```python
from build123d import *

# Parameters (mm, degrees)
SKETCH_2_W                  = 47
SKETCH_2_H                  = 47
EXTRUDE_1_DEPTH             = 4
SKETCH_3_W                  = 47
SKETCH_3_H                  = 2
EXTRUDE_2_DEPTH             = 43
SKETCH_4_W                  = 4
SKETCH_4_H                  = 45
EXTRUDE_3_DEPTH             = 43
SKETCH_5_R                  = 12.5
CUT_EXTRUDE_1_DEPTH         = 81.268300094
M3X0_5_2_D                  = 3
HOLE_WIZARD_M5_1_AT_2_COUNT = 2
HOLE_WIZARD_M5_1_AT_2_PITCH = 14.142135624
HOLE_WIZARD_M5_1_AT_3_COUNT = 2
HOLE_WIZARD_M5_1_AT_3_PITCH = 20
HOLE_WIZARD_M5_1_AT_4_COUNT = 2
HOLE_WIZARD_M5_1_AT_4_PITCH = 14.142135624
EXTRUDE_6_DEPTH             = 45
EXTRUDE_7_DEPTH             = 45
SKETCH_23_W                 = 67
SKETCH_23_H                 = 47
SKETCH_23_R                 = 3.5
SKETCH_23_R_2               = 12.5
EXTRUDE_10_DEPTH            = 3
M2X0_4_1_D                  = 2
SKETCH_27_W                 = 47
SKETCH_27_H                 = 1
CUT_EXTRUDE_2_DEPTH         = 20
FILLET_1_R                  = 2.5
FILLET_2_R                  = 4
SKETCH_29_W                 = 47
SKETCH_29_H                 = 2
EXTRUDE_11_DEPTH            = 20
FILLET_5_R                  = 4
FILLET_6_R                  = 3
M2X0_4_2_D                  = 2
SKETCH_34_W                 = 20
SKETCH_34_H                 = 47
CUT_EXTRUDE_5_DEPTH         = 20
FILLET_7_R                  = 4


with BuildPart() as part:
    # ｽｹｯﾁ2 → ﾎﾞｽ - 押し出し1 (new body)
    with BuildSketch(Plane.XY):
        with Locations((23.5, 23.5)):
            Rectangle(SKETCH_2_W, SKETCH_2_H)
    extrude(amount=EXTRUDE_1_DEPTH)

    # ｽｹｯﾁ3 → ﾎﾞｽ - 押し出し2 (add)
    with BuildSketch(Plane.XY.offset(4)):
        with Locations((23.5, 46)):
            Rectangle(SKETCH_3_W, SKETCH_3_H)
    extrude(amount=EXTRUDE_2_DEPTH)

    # ｽｹｯﾁ4 → ﾎﾞｽ - 押し出し3 (add)
    with BuildSketch(Plane.XY.offset(4)):
        with Locations((45, 22.5)):
            Rectangle(SKETCH_4_W, SKETCH_4_H)
    extrude(amount=EXTRUDE_3_DEPTH)

    # ｽｹｯﾁ5 → ｶｯﾄ - 押し出し1 (cut, through all)
    with BuildSketch(Plane.XZ.offset(-45)):
        with Locations(Location((21.5, 25.5, 0), (0, 0, 270))):
            Circle(SKETCH_5_R)
    extrude(amount=-CUT_EXTRUDE_1_DEPTH, mode=Mode.SUBTRACT)

    # M3x0.5 ねじ穴2 (through all)
    with Locations(Plane(origin=(0, 47, 0), x_dir=(1, 0, 0), z_dir=(0, 1, 0))):
        with Locations((6, -10), (37, -10), (37, -41), (6, -41)):
            Hole(M3X0_5_2_D / 2)

    # ｽｹｯﾁ14 → M5 平皿頭ねじ用皿穴1 (revolve, cut)
    with BuildSketch(Plane(origin=(11.5, 22, 4), x_dir=(0, -1, 0), z_dir=(1, 0, 0))):
        Polygon((0, 0), (0, 4), (2.75, 4), (2.75, 2.45), (5.2, 0), align=None)
    hole_wizard_m5_1 = revolve(axis=Axis((11.5, 22, 10.35), (0, 0, -1)), mode=Mode.SUBTRACT)

    # M5 平皿頭ねじ用皿穴1 at 2: M5 平皿頭ねじ用皿穴1 ×2
    with Locations(*[Vector(0.7071067811865475, 0.7071067811865476, 0) * (i * HOLE_WIZARD_M5_1_AT_2_PITCH) for i in range(1, HOLE_WIZARD_M5_1_AT_2_COUNT)]):
        add(hole_wizard_m5_1, mode=Mode.SUBTRACT)

    # M5 平皿頭ねじ用皿穴1 at 3: M5 平皿頭ねじ用皿穴1 ×2
    with Locations(*[(i * HOLE_WIZARD_M5_1_AT_3_PITCH, 0, 0) for i in range(1, HOLE_WIZARD_M5_1_AT_3_COUNT)]):
        add(hole_wizard_m5_1, mode=Mode.SUBTRACT)

    # M5 平皿頭ねじ用皿穴1 at 4: M5 平皿頭ねじ用皿穴1 ×2
    with Locations(*[Vector(0.7071067811865474, -0.7071067811865478, 0) * (i * HOLE_WIZARD_M5_1_AT_4_PITCH) for i in range(1, HOLE_WIZARD_M5_1_AT_4_COUNT)]):
        add(hole_wizard_m5_1, mode=Mode.SUBTRACT)

    # ｽｹｯﾁ17 → ﾎﾞｽ - 押し出し6 (add)
    with BuildSketch(Plane.XZ.offset(-45)):
        Polygon((43, 4), (39.5, 4), (43, 7.5), align=None)
    extrude(amount=EXTRUDE_6_DEPTH)

    # ｽｹｯﾁ19 → ﾎﾞｽ - 押し出し7 (add)
    with BuildSketch(Plane.XZ.offset(-45)):
        Polygon((0, 4), (3.5, 4), (0, 7.5), align=None)
    extrude(amount=EXTRUDE_7_DEPTH)

    # ｽｹｯﾁ23 → ﾎﾞｽ - 押し出し10 (add)
    with BuildSketch(Plane(origin=(0, 47, 0), x_dir=(1, 0, 0), z_dir=(0, 1, 0))):
        with Locations((13.5, -23.5)):
            Rectangle(SKETCH_23_W, SKETCH_23_H)
        with Locations(Location((6, -10, 0), (0, 0, 270))):
            Circle(SKETCH_23_R, mode=Mode.SUBTRACT)
        with Locations(Location((6, -41, 0), (0, 0, 270))):
            Circle(SKETCH_23_R, mode=Mode.SUBTRACT)
        with Locations(Location((37, -10, 0), (0, 0, 270))):
            Circle(SKETCH_23_R, mode=Mode.SUBTRACT)
        with Locations(Location((37, -41, 0), (0, 0, 270))):
            Circle(SKETCH_23_R, mode=Mode.SUBTRACT)
        with Locations(Location((21.5, -25.5, 0), (0, 0, 90))):
            Circle(SKETCH_23_R_2, mode=Mode.SUBTRACT)
    extrude(amount=EXTRUDE_10_DEPTH)

    # M2x0.4 ねじ穴1 (through all)
    with Locations(Plane(origin=(0, 50, 0), x_dir=(1, 0, 0), z_dir=(0, 1, 0))):
        with Locations((-5, -18), (-14.5, -18)):
            Hole(M2X0_4_1_D / 2)

    # ｽｹｯﾁ27 → ｶｯﾄ - 押し出し2 (cut)
    with BuildSketch(Plane.ZY.offset(20)):
        with Locations((23.5, 47.5)):
            Rectangle(SKETCH_27_W, SKETCH_27_H)
    extrude(amount=-CUT_EXTRUDE_2_DEPTH, mode=Mode.SUBTRACT)

    # ﾌｨﾚｯﾄ1
    fillet_1_edges = [part.edges().sort_by_distance(p)[0] for p in [
        (0, 48, 23.5),
    ]]
    fillet(fillet_1_edges, radius=FILLET_1_R)

    # ﾌｨﾚｯﾄ2
    fillet_2_edges = [part.edges().sort_by_distance(p)[0] for p in [
        (-20, 49, 47),
        (-20, 49, 0),
        (0, 0, 3.75),
        (45, 0, 47),
    ]]
    fillet(fillet_2_edges, radius=FILLET_2_R)

    # ｽｹｯﾁ29 → ﾎﾞｽ - 押し出し11 (add)
    with BuildSketch(Plane(origin=(47, 0, 0), x_dir=(0, 0, -1), z_dir=(1, 0, 0))):
        with Locations((-23.5, 49)):
            Rectangle(SKETCH_29_W, SKETCH_29_H)
    extrude(amount=EXTRUDE_11_DEPTH)

    # ﾌｨﾚｯﾄ5
    fillet_5_edges = [part.edges().sort_by_distance(p)[0] for p in [
        (67, 49, 0),
        (67, 49, 47),
    ]]
    fillet(fillet_5_edges, radius=FILLET_5_R)

    # ﾌｨﾚｯﾄ6
    fillet_6_edges = [part.edges().sort_by_distance(p)[0] for p in [
        (47, 48, 23.5),
    ]]
    fillet(fillet_6_edges, radius=FILLET_6_R)

    # M2x0.4 ねじ穴2 (through all)
    with Locations(Plane(origin=(0, 50, 0), x_dir=(1, 0, 0), z_dir=(0, 1, 0))):
        with Locations((61.5, -18), (52, -18)):
            Hole(M2X0_4_2_D / 2)

    # ｽｹｯﾁ34 → ｶｯﾄ - 押し出し5 (cut)
    with BuildSketch(Plane(origin=(0, 50, 0), x_dir=(1, 0, 0), z_dir=(0, 1, 0))):
        with Locations((-10, -23.5)):
            Rectangle(SKETCH_34_W, SKETCH_34_H)
    extrude(amount=-CUT_EXTRUDE_5_DEPTH, mode=Mode.SUBTRACT)

    # ﾌｨﾚｯﾄ7
    fillet_7_edges = [part.edges().sort_by_distance(p)[0] for p in [
        (0, 47.5, 47),
    ]]
    fillet(fillet_7_edges, radius=FILLET_7_R)


solid = part.part
```
The model under review builds one solid part; all positions refer to its coordinate system, in mm. A direction names the side the tool comes from. Round coordinates to 2 decimals unless told otherwise and drop trailing zeros. Write each loop counter-clockwise with the first axis right and the second up, starting at its lowest first coordinate (ties: lowest second). Pieces come first, ordered by that corner, then holes.
(1) We need section C-C on y = 22. Give the boundary of the cut face in (x, z), and give its area (3 significant figures).
(2) Insertion check: pin 1 (10 mm diameter, centred on x = 32, y = 14.5, fed in from +Z); pin 2 (8 mm diameter, centred on y = 34.5, z = 10.5, fed in from +X); pin 3 (2 mm diameter, centred on x = 6.5, z = 10.5, fed in from +Y); pin 4 (4.5 mm diameter, centred on x = 11.5, y = 22, fed in from +Z). Each pin has a flat end and moves straight along its axis. Give the tip position at first contact, or say it passes through.
(3) We need section B-B on x = 31.5. Give the boundary of the cut face in (y, z).
(4) We need section A-A on z = 25. Give the boundary of the cut face in (x, y), and give its area (3 significant figures).
(5) We need section D-D on z = 10. Give the boundary of the cut face in (x, y), and give its area (3 significant figures).
(6) Mouldability with a two-part tool opening along X and no side actions: class faces 1 (the conical face through (14.33, 22.63, 1.7)), 2 (the flat face through (43, 22, 27)), 3 (the cylindrical face through (65.797, 49.014, 45.859)) as +X half, -X half, draft (parallel to the pull), parting line (faces both ways), or undercut.
(7) Machinability: for faces 4 (the flat face through (21, 23, 4)), 5 (the flat face through (37, 47, 12)), 6 (the conical face through (28.621, 22.378, 1.703)), which of the approach directions +Z, -Z, +X, -X, +Y, -Y give a long, thin tool a straight path to every point of the face, cutting with its end or side? Answer none if there is none.
(8) Wall thickness on L1, parallel to Z at x = 6, y = 45.95; L2, parallel to X at y = 46.5, z = 41; L3, parallel to X at y = 5.5, z = 5: over which ranges is each line inside the solid? List them lowest first.
Findings below:
1. outline: (0, 0) - (8.75, 0) - (8.75, 1.55) - (6.3, 4) - (3.5, 4) - (0, 7.5) - close; (14.25, 0) - (28.75, 0) - (28.75, 1.55) - (26.3, 4) - (16.7, 4) - (14.25, 1.55) - close; (34.25, 0) - (47, 0) - (47, 47) - (43, 47) - (43, 7.5) - (39.5, 4) - (36.7, 4) - (34.25, 1.55) - close
1. area: 316 mm2
2. pin 1: stops at z = 4
2. pin 2: stops at x = 47
2. pin 3: stops at y = 47
2. pin 4: passes through
3. outline: (0, 0) - (19.25, 0) - (19.25, 1.55) - (16.8, 4) - (0, 4) - close; (24.75, 0) - (50, 0) - (50, 18) - (45, 18) - (45, 4) - (27.2, 4) - (24.75, 1.55) - close; (45, 33) - (50, 33) - (50, 47) - (45, 47) - close
4. outline: (0, 45) - (9.01, 45) - (9.01, 50) - (0, 50) - close; (33.99, 45) - (43, 45) - (43, 0) - (47, 0) - (47, 45) arc R3 cw to (50, 48) - (67, 48) - (67, 50) - (33.99, 50) - close
4. area: 332 mm2
5. outline: (0, 45) - (4.5, 45) - (4.5, 47) - (2.5, 47) - (2.5, 50) - (0, 50) - close; (7.5, 45) - (35.5, 45) - (35.5, 47) - (33.5, 47) - (33.5, 50) - (9.5, 50) - (9.5, 47) - (7.5, 47) - close; (38.5, 45) - (43, 45) - (43, 0) - (47, 0) - (47, 45) arc R3 cw to (50, 48) - (67, 48) - (67, 50) - (40.5, 50) - (40.5, 47) - (38.5, 47) - close
5. area: 403 mm2
6. face 1: undercut
6. face 2: -X half
6. face 3: +X half
7. face 4: +Z, -Y
7. face 5: +Y
7. face 6: +Z
8. L1: z = 0 to 8.5, 11.5 to 39.5, 42.5 to 47
8. L2: x = 0 to 4.5, 7.5 to 35.5, 38.5 to 47.4
8. L3: x = 0 to 2.5, 40.5 to 47
